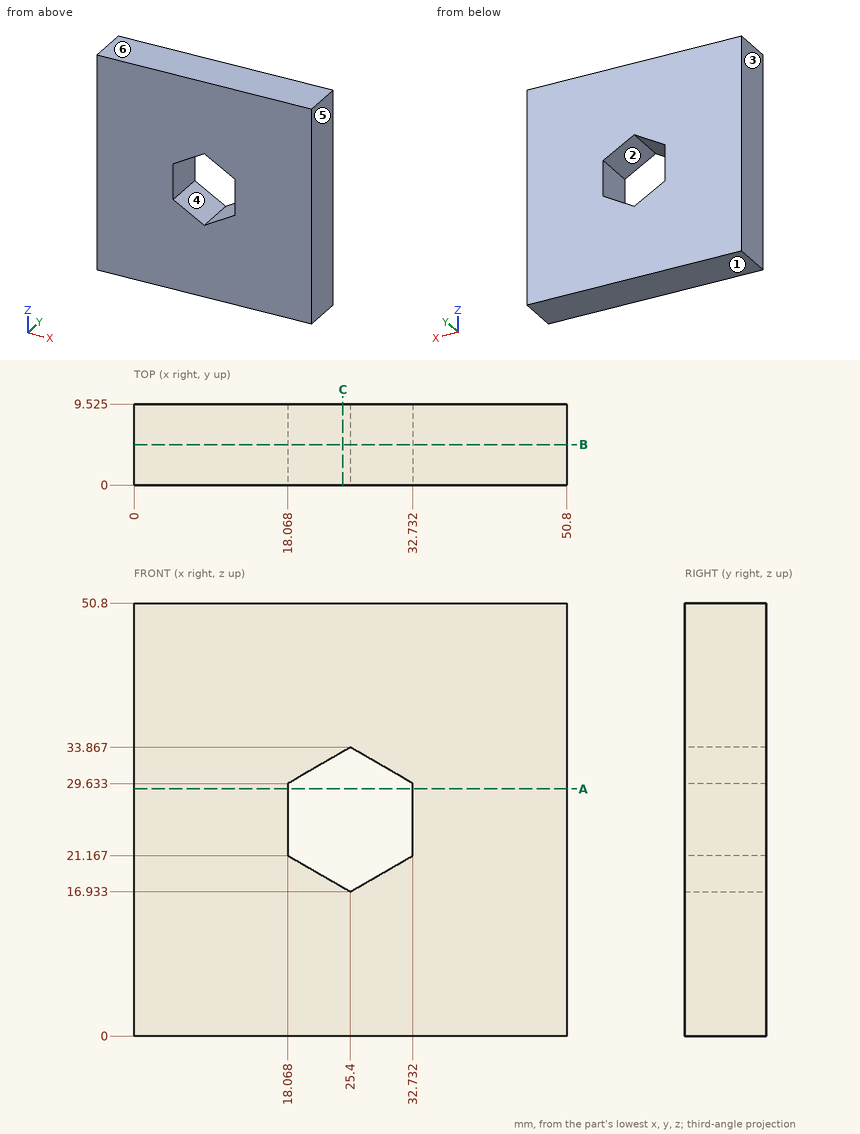
Verification items for this drawing (mm, ordinates from the low corner). A direction names the side the tool comes from. Round coordinates to 2 decimals unless told otherwise and drop trailing zeros. Write each loop counter-clockwise with the first axis right and the second up, starting at its lowest first coordinate (ties: lowest second). Pieces come first, ordered by that corner, then holes. Notation, with made-up numbers: (-9.5, -9) - (40.5, -9) arc R27 ccw to (40.5, 8) - close; hole circle Ø3 at (35, -17.5). An arc over 180 degrees is marked (long way). One line per item, written item: value.
1. Mould release check, pull along X, two halves, no side actions. Record for the marked faces 3, 4, 5 and 6: released by +X, released by -X, zero draft, split by the parting line, or undercut.
The answers:
face 3: released by -X
face 4: undercut
face 5: released by +X
face 6: zero draft
2. Cross-section at B-B on y = 4.75. Record the boundary of the cut face in (x, z), and give its area (3 significant figures).
The answers:
outline: (0, 0) - (50.8, 0) - (50.8, 50.8) - (0, 50.8) - close; hole (18.07, 21.17) - (25.4, 16.93) - (32.73, 21.17) - (32.73, 29.63) - (25.4, 33.87) - (18.07, 29.63) - close
area: 2,390 mm^2
3. Cross-section at C-C on x = 24.5. Record the boundary of the cut face in (y, z) (1 decimal).
The answers:
outline: (0, 0) - (9.5, 0) - (9.5, 17.5) - (0, 17.5) - close; (0, 33.3) - (9.5, 33.3) - (9.5, 50.8) - (0, 50.8) - close
4. Set-up check for the marked faces 1 and 2: record each of +Z, -Z, +X, -X, +Y, -Y from which the full face is reachable in a straight line by a thin tool's end or side.
The answers:
face 1: -Z, +X, -X, +Y, -Y
face 2: +Y, -Y
5. Cross-section at A-A on z = 29. Record the boundary of the cut face in (x, y) (1 decimal), and give its area (3 significant figures).
The answers:
outline: (0, 0) - (18.1, 0) - (18.1, 9.5) - (0, 9.5) - close; (32.7, 0) - (50.8, 0) - (50.8, 9.5) - (32.7, 9.5) - close
area: 344 mm^2
6. Scan lines: L1, parallel to Z at x = 24.5, y = 2.25; L2, parallel to Z at x = 32.5, y = 0.75. Record each from-to range of solid material in increasing order.
The answers:
L1: z = 0 to 17.45, 33.35 to 50.8
L2: z = 0 to 21.03, 29.77 to 50.8
